The drawing under review shows one solid part. Ordinate dimensions are in mm from its lowest x, y, z. A direction names the side the tool comes from. Coordinates: 2 decimals unless noted, no trailing zeros. Order: outer loops, then holes, each group sorted by start corner. A loop starts at its lowest first (then second) coordinate and runs counter-clockwise, first axis right, second up.
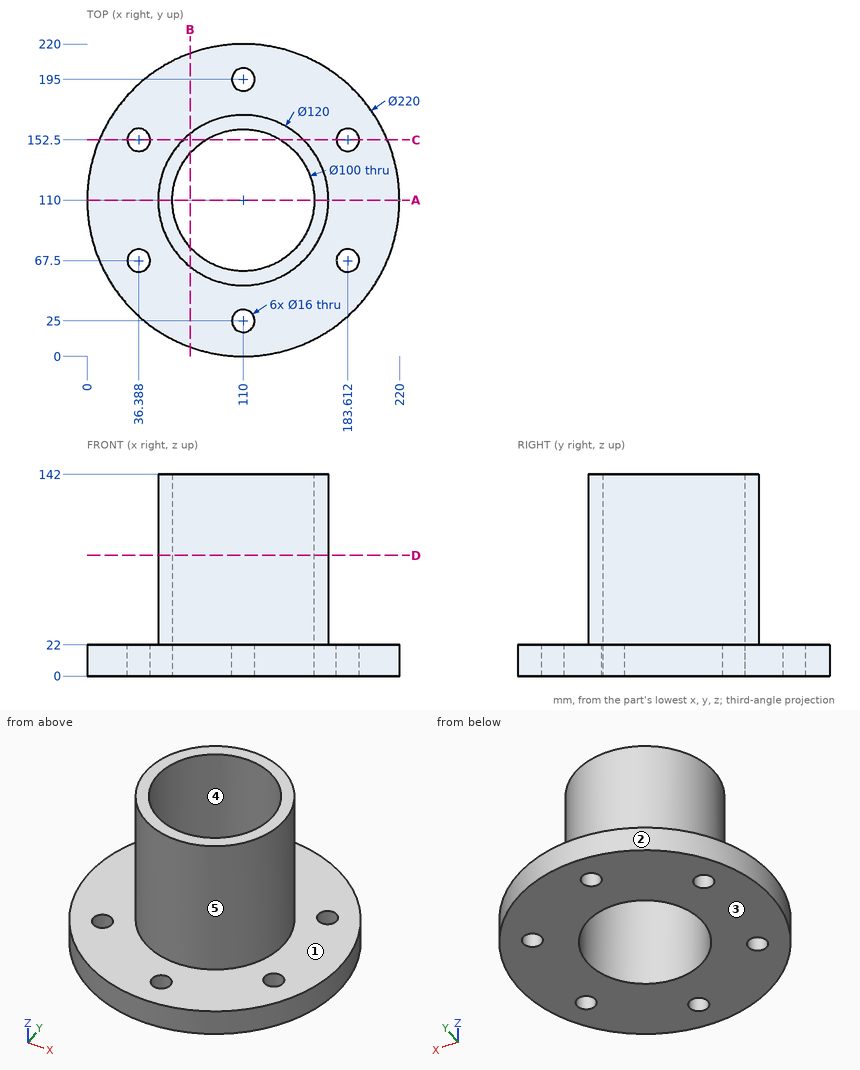
1. Mouldability with a two-part tool opening along X and no side actions: class the marked faces 3, 4 and 5 as pulls with the +X half, pulls with the -X half, needs draft (parallel to the pull), parting line crosses it, or undercut.
2. Insertion check: pin 1 (8 mm diameter, centred on x = 81.5, z = 87.5, fed in from +Y); pin 2 (1.5 mm diameter, centred on x = 88.5, y = 189, fed in from +Z); pin 3 (5 mm diameter, centred on y = 73, z = 49.5, fed in from +X). Each pin has a flat end and moves straight along its axis. Give the tip position at first contact, or say it passes through.
3. Add section D-D (z = 85). Give the boundary of the cut face in (x, y), and give its area (3 significant figures).
4. Add section A-A (y = 110). Give the boundary of the cut face in (x, z), and give its area (3 significant figures).
5. Add section B-B (x = 72.5). Give the boundary of the cut face in (y, z).
6. For the marked faces 1 and 2, list the 3-axis set-ups (+Z, -Z, +X, -X, +Y, -Y) from which the entire face can be reached by the end or side of a thin tool; tool diameter is ignored.
7. Add section C-C (y = 152.5). Give the boundary of the cut face in (x, z).
8. To check wall thickness, follow line 1 (Y direction, x = 110, z = 5); line 2 (X direction, y = 152, z = 9) (1 decimal); line 3 (Y direction, x = 110, z = 43). State the ranges of each line that lie inside material, in increasing order.
Solution:
1. face 3: needs draft
1. face 4: undercut
1. face 5: parting line crosses it
2. pin 1: stops at y = 164.77
2. pin 2: stops at z = 22
2. pin 3: stops at x = 159.09
3. outline: circle Ø120 at (110, 110); hole circle Ø100 at (110, 110)
3. area: 3,460 mm2
4. outline: (0, 0) - (60, 0) - (60, 142) - (50, 142) - (50, 22) - (0, 22) - close; (160, 0) - (220, 0) - (220, 22) - (170, 22) - (170, 142) - (160, 142) - close
4. area: 5,040 mm2
5. outline: (6.59, 0) - (76.93, 0) - (76.93, 142) - (63.16, 142) - (63.16, 22) - (6.59, 22) - close; (143.07, 0) - (213.41, 0) - (213.41, 22) - (156.84, 22) - (156.84, 142) - (143.07, 142) - close
6. face 1: +Z
6. face 2: +Z, -Z
7. outline: (8.54, 0) - (28.39, 0) - (28.39, 22) - (8.54, 22) - close; (44.39, 0) - (83.66, 0) - (83.66, 142) - (67.65, 142) - (67.65, 22) - (44.39, 22) - close; (136.34, 0) - (175.61, 0) - (175.61, 22) - (152.35, 22) - (152.35, 142) - (136.34, 142) - close; (191.61, 0) - (211.46, 0) - (211.46, 22) - (191.61, 22) - close
8. line 1: y = 0 to 17, 33 to 60, 160 to 187, 203 to 220
8. line 2: x = 8.3 to 28.4, 44.4 to 82.9, 137.1 to 175.6, 191.6 to 211.7
8. line 3: y = 50 to 60, 160 to 170
